Input: part model. Units: mm. Frame: model coordinates. Round coordinates to 2 decimals unless told otherwise and drop trailing zeros. Write each loop counter-clockwise with the first axis right and the second up, starting at its lowest first coordinate (ties: lowest second). Pieces come first, ordered by that corner, then holes. Notation, with made-up numbers: (70, 28) -> (77, 28) arc R29 cw to (77, 50) -> close; hole circle Ø3 at (-27, -11.75). An arc over 180 degrees is marked (long way). Use CSV: the item, a comma, the result in double quotes.
```python
from build123d import *

# Parameters (mm, degrees)
F0_R     = 30
F1_DEPTH = 10
F2_D     = 11


with BuildPart() as f1:
    # F0 (on Front) → F1 (new body)
    with BuildSketch(Plane.XZ):
        with BuildLine():
            ThreePointArc((55, 23), (51.485281, 31.485281), (43, 35))
            Line((43, 35), (-43, 35))
            ThreePointArc((-43, 35), (-51.485281, 31.485281), (-55, 23))
            Line((-55, 23), (-55, -23))
            ThreePointArc((-55, -23), (-51.485281, -31.485281), (-43, -35))
            Line((-43, -35), (43, -35))
            ThreePointArc((43, -35), (51.485281, -31.485281), (55, -23))
            Line((55, -23), (55, 23))
        make_face()
        Circle(F0_R, mode=Mode.SUBTRACT)
    extrude(amount=F1_DEPTH)

    # F2 (through all)
    with Locations(Plane(origin=(0, 0, 0), x_dir=(1, 0, 0), z_dir=(0, 1, 0))):
        with Locations((-41, 24), (41, 24), (41, -24), (-41, -24)):
            Hole(F2_D / 2)


solid = f1.part
```
Item 1: Section query B-B on x = 41. Return the cut outline in (y, z), plus the area to 3 significant figures.
Worked answers:
outline,"(-10, -35) -> (0, -35) -> (0, -29.5) -> (-10, -29.5) -> close; (-10, -18.5) -> (0, -18.5) -> (0, 18.5) -> (-10, 18.5) -> close; (-10, 29.5) -> (0, 29.5) -> (0, 35) -> (-10, 35) -> close"
area,"480 mm²"
Item 2: Line query: line 1 (Z direction, x = -41, y = -5.5); line 2 (X direction, y = -1, z = -5.5); line 3 (Z direction, x = -37, y = -3). Output: solid intervals per line, ascending.
Worked answers:
line 1,"z = -35 to -29.5, -18.5 to 18.5, 29.5 to 35"
line 2,"x = -55 to -29.49, 29.49 to 55"
line 3,"z = -35 to -27.77, -20.23 to 20.23, 27.77 to 35"
Item 3: Pull-direction query (X, two-part tool) for faces 1 (the face through (-1, -5, -35)), 2 (the face through (-51.39, -4.93, 31.58)), 3 (the face through (-35.505, -5.07, -24.242)); classes: +X half, -X half, draft (parallel to the pull), parting line (faces both ways), or undercut.
Worked answers:
face 1,"draft"
face 2,"-X half"
face 3,"undercut"
Item 4: Section query C-C on z = 0. Return the cut outline in (x, y), plus the area to 3 significant figures.
Worked answers:
outline,"(-55, -10) -> (-30, -10) -> (-30, 0) -> (-55, 0) -> close; (30, -10) -> (55, -10) -> (55, 0) -> (30, 0) -> close"
area,"500 mm²"
Item 5: Section query A-A on y = -2.25. Return the cut outline in (x, z), plus the area to 3 significant figures.
Worked answers:
outline,"(-55, -23) arc R12 ccw to (-43, -35) -> (43, -35) arc R12 ccw to (55, -23) -> (55, 23) arc R12 ccw to (43, 35) -> (-43, 35) arc R12 ccw to (-55, 23) -> close; hole circle Ø11 at (-41, -24); hole circle Ø11 at (-41, 24); hole circle Ø60 at (0, 0); hole circle Ø11 at (41, -24); hole circle Ø11 at (41, 24)"
area,"4,370 mm²"
Item 6: Section query D-D on x = 0. Return the cut outline in (y, z), plus the area to 3 significant figures.
Worked answers:
outline,"(-10, -35) -> (0, -35) -> (0, -30) -> (-10, -30) -> close; (-10, 30) -> (0, 30) -> (0, 35) -> (-10, 35) -> close"
area,"100 mm²"
